Read the model definition and answer for the solid it produces. Units are mm, in the model's axes. Face numbers are marked on the shaded views. A direction names the side the tool comes from. Coordinates: 2 decimals unless noted, no trailing zeros. Write each loop counter-clockwise with the first axis right and the second up, starting at its lowest first coordinate (ties: lowest second). Pieces come first, ordered by that corner, then holes.
1) Determine the mould class of the marked faces 1, 2, 3 and 4 for opening direction Z: +Z half, -Z half, draft (parallel to the pull), parting line (faces both ways), or undercut.
2) The part is cut by section A-A (x = 21). Determine the outline of the cut face in (y, z) (3 decimals).
3) Which of the six approach directions +Z, -Z, +X, -X, +Y, -Y give full straight-line access (tool end or side, diameter ignored) to the marked faces 5 and 6?
4) The part is cut by section D-D (z = -21). Determine the outline of the cut face in (x, y), then the cut area to 3 significant figures.
5) Find the intervals of material crossed by line 1 (X direction, y = 3.25, z = -21.5); line 2 (Z direction, x = 21.5, y = 4); line 3 (Z direction, x = 31, y = 2), in increasing order.
6) The part is cut by section C-C (y = 19.25). Determine the outline of the cut face in (x, z) (3 decimals), then the cut area to 3 significant figures.
7) Each of these flat-tipped pins is pushed along its axis until it touches: pin 1 Ø1 at (x, z) = (22.5, -21.5) entering from +Y; pin 2 Ø10 at (x, z) = (19.5, -21) entering from -Y; pin 3 Ø5 at (x, z) = (37, -37.5) entering from -Y. Where does it stop, or does it pass through?
8) The part is cut by section B-B (y = 9). Determine the outline of the cut face in (x, z) (3 decimals).
from build123d import *

# Parameters (mm, degrees)
SKETCH1_W           = 42
SKETCH1_H           = 42
BOSS_EXTRUDE1_DEPTH = 20.75
SKETCH2_W           = 9.5
SKETCH2_H           = 3.5
CUT_EXTRUDE4_DEPTH  = 3.52
SKETCH3_W           = 15.5
SKETCH3_H           = 10.5
CUT_EXTRUDE1_DEPTH  = 15.23
CUT_EXTRUDE2_REACH  = 19.23
SKETCH5_W           = 34
SKETCH5_H           = 34
SKETCH5_W_2         = 21.5
SKETCH5_H_2         = 16.5
CUT_EXTRUDE5_DEPTH  = 10
FILLET1_R           = 3.175


with BuildPart() as part:
    # Sketch1 → Boss-Extrude1 (new body)
    with BuildSketch(Plane(origin=(0, 0, 0), x_dir=(1, 0, 0), z_dir=(0, 1, 0))):
        with Locations((21, 21)):
            Rectangle(SKETCH1_W, SKETCH1_H)
    extrude(amount=BOSS_EXTRUDE1_DEPTH)

    # Sketch2 → Cut-Extrude4 (cut)
    with BuildSketch(Plane(origin=(0, 20.75, 0), x_dir=(1, 0, 0), z_dir=(0, 1, 0))):
        with Locations((21, 21)):
            Rectangle(SKETCH2_W, SKETCH2_H)
    extrude(amount=-CUT_EXTRUDE4_DEPTH, mode=Mode.SUBTRACT)

    # Sketch3 → Cut-Extrude1 (cut)
    with BuildSketch(Plane.XZ):
        with Locations((21, -21)):
            Rectangle(SKETCH3_W, SKETCH3_H)
    extrude(amount=-CUT_EXTRUDE1_DEPTH, mode=Mode.SUBTRACT)

    # Sketch4 → Cut-Extrude2 (cut, up to next)
    with BuildSketch(Plane(origin=(0, 17.23, 0), x_dir=(1, 0, 0), z_dir=(0, 1, 0)), mode=Mode.PRIVATE) as cut_extrude2_sk1:
        with BuildLine():
            Line((17.975, 22.275), (24.025, 22.275))
            ThreePointArc((24.025, 22.275), (25.3, 21), (24.025, 19.725))
            Line((24.025, 19.725), (17.975, 19.725))
            ThreePointArc((17.975, 19.725), (16.7, 21), (17.975, 22.275))
        make_face()
    cut_extrude2_tool1 = extrude(cut_extrude2_sk1.sketch, amount=-CUT_EXTRUDE2_REACH, mode=Mode.PRIVATE) & part.part
    add(cut_extrude2_tool1.solids().sort_by_distance((21, 17.23, -21))[0], mode=Mode.SUBTRACT)

    # Sketch5 → Cut-Extrude5 (cut)
    with BuildSketch(Plane.XZ):
        with Locations((21, -21)):
            Rectangle(SKETCH5_W, SKETCH5_H)
        with Locations((21, -21)):
            Rectangle(SKETCH5_W_2, SKETCH5_H_2, mode=Mode.SUBTRACT)
    extrude(amount=-CUT_EXTRUDE5_DEPTH, mode=Mode.SUBTRACT)

    # Fillet1
    fillet1_edges = [part.edges().sort_by_distance(p)[0] for p in [
        (0, 10.375, -42),
        (42, 10.375, -42),
        (42, 10.375, 0),
        (0, 10.375, 0),
    ]]
    fillet(fillet1_edges, radius=FILLET1_R)


solid = part.part
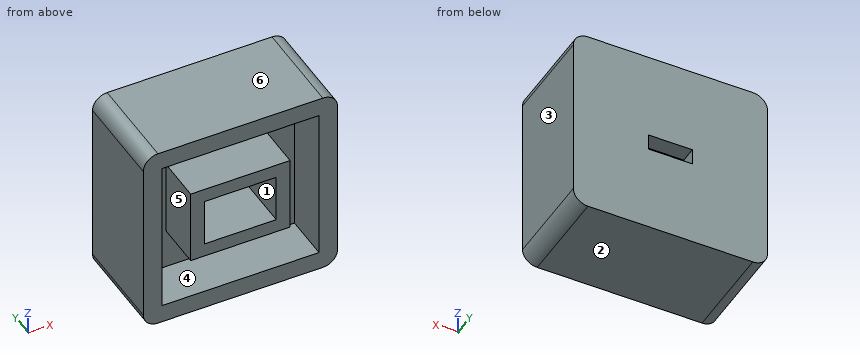
Reported:
1. face 1: undercut
1. face 2: -Z half
1. face 3: draft
1. face 4: undercut
2. outline: (0, -42) - (20.75, -42) - (20.75, -22.75) - (17.23, -22.75) - (17.23, -22.275) - (15.23, -22.275) - (15.23, -26.25) - (0, -26.25) - (0, -29.25) - (10, -29.25) - (10, -38) - (0, -38) - close; (0, -15.75) - (15.23, -15.75) - (15.23, -19.725) - (17.23, -19.725) - (17.23, -19.25) - (20.75, -19.25) - (20.75, 0) - (0, 0) - (0, -4) - (10, -4) - (10, -12.75) - (0, -12.75) - close
3. face 5: -Y
3. face 6: +Z, +X, -X, +Y, -Y
4. outline: (0, 0) - (4, 0) - (4, 10) - (10.25, 10) - (10.25, 0) - (13.25, 0) - (13.25, 15.23) - (16.7, 15.23) - (16.7, 17.23) - (16.25, 17.23) - (16.25, 20.75) - (0, 20.75) - close; (25.3, 15.23) - (28.75, 15.23) - (28.75, 0) - (31.75, 0) - (31.75, 10) - (38, 10) - (38, 0) - (42, 0) - (42, 20.75) - (25.75, 20.75) - (25.75, 17.23) - (25.3, 17.23) - close
4. area: 460 mm2
5. line 1: x = 0 to 4, 10.25 to 13.25, 28.75 to 31.75, 38 to 42
5. line 2: z = -42 to -38, -29.25 to -26.25, -15.75 to -12.75, -4 to 0
5. line 3: z = -42 to -38, -29.25 to -12.75, -4 to 0
6. outline: (0, -38.825) arc R3.175 ccw to (3.175, -42) - (38.825, -42) arc R3.175 ccw to (42, -38.825) - (42, -3.175) arc R3.175 ccw to (38.825, 0) - (3.175, 0) arc R3.175 ccw to (0, -3.175) - close; hole (16.25, -22.75) - (25.75, -22.75) - (25.75, -19.25) - (16.25, -19.25) - close
6. area: 1,720 mm2
7. pin 1: passes through
7. pin 2: stops at y = 15.23
7. pin 3: stops at y = 0
8. outline: (0, -38.825) arc R3.175 ccw to (3.175, -42) - (38.825, -42) arc R3.175 ccw to (42, -38.825) - (42, -3.175) arc R3.175 ccw to (38.825, 0) - (3.175, 0) arc R3.175 ccw to (0, -3.175) - close; (10.25, -29.25) - (31.75, -29.25) - (31.75, -12.75) - (10.25, -12.75) - close; hole (4, -38) - (38, -38) - (38, -4) - (4, -4) - close; hole (13.25, -26.25) - (28.75, -26.25) - (28.75, -15.75) - (13.25, -15.75) - close
